Could you check a few things on this model? Use its own coordinates, in mm. A direction names the side the tool comes from. Round coordinates to 2 decimals unless told otherwise and drop trailing zeros. Write each loop counter-clockwise with the first axis right and the second up, starting at its lowest first coordinate (ties: lowest second). Pieces come first, ordered by that corner, then holes. Notation, with made-up numbers: (31, 89) -> (69, 89) arc R15 cw to (69, 104) -> close; hole circle Ø3 at (21, 45). An arc over 180 degrees is marked (long way). Answer in a Markdown table with one row per item. Add a question column.
```python
from build123d import *

# Parameters (mm, degrees)
SKETCH1_W                      = 75.565
SKETCH1_H                      = 35.56
BOSS_EXTRUDE1_DEPTH            = 3.175
SKETCH5_W                      = 12.7
SKETCH5_H                      = 3.175
BOSS_EXTRUDE3_DEPTH            = 14.986
SKETCH6_W                      = 3.175
SKETCH6_H                      = 9.028368652
BOSS_EXTRUDE4_DEPTH            = 14.986
BOSS_EXTRUDE5_DEPTH            = 12.7
BOSS_EXTRUDE6_DEPTH            = 9.028368652
BOSS_EXTRUDE7_DEPTH            = 75.565
SKETCH10_W                     = 75.565
SKETCH10_H                     = 23.368
BOSS_EXTRUDE8_DEPTH            = 5.08
CUT_EXTRUDE1_DEPTH             = 82.106081899
CUT_EXTRUDE2_REACH             = 52.218
SKETCH12_W                     = 6.35
SKETCH12_H                     = 3.175
CUT_EXTRUDE2_DIRECTION_2_DEPTH = 51.217629864
CUT_EXTRUDE3_DEPTH             = 55.104465738
CUT_EXTRUDE4_REACH             = 55.629
SKETCH14_W                     = 2.54
SKETCH14_H                     = 3.81


with BuildPart() as part:
    # Sketch1 → Boss-Extrude1 (new body)
    with BuildSketch(Plane.XY):
        Rectangle(SKETCH1_W, SKETCH1_H)
    extrude(amount=-BOSS_EXTRUDE1_DEPTH)

    # Sketch5 → Boss-Extrude3 (add)
    with BuildSketch(Plane.XY):
        with Locations((0, 16.1925)):
            Rectangle(SKETCH5_W, SKETCH5_H)
        with Locations((0, -16.1925)):
            Rectangle(SKETCH5_W, SKETCH5_H)
    extrude(amount=BOSS_EXTRUDE3_DEPTH)

    # Sketch6 → Boss-Extrude4 (add)
    with BuildSketch(Plane.XY):
        with Locations((-36.195, 0)):
            Rectangle(SKETCH6_W, SKETCH6_H)
        with Locations((36.195, 0)):
            Rectangle(SKETCH6_W, SKETCH6_H)
    extrude(amount=BOSS_EXTRUDE4_DEPTH)

    # Sketch7 → Boss-Extrude5 (add)
    with BuildSketch(Plane.ZY.offset(6.35)):
        Polygon((14.986, -17.78), (14.986, -11.43), (21.336, -17.78), align=None)
        Polygon((14.986, 17.78), (14.986, 11.43), (21.336, 17.78), align=None)
    extrude(amount=-BOSS_EXTRUDE5_DEPTH)

    # Sketch8 → Boss-Extrude6 (add)
    with BuildSketch(Plane.XZ.offset(4.514184326)):
        Polygon((-37.7825, 14.986), (-31.4325, 14.986), (-37.7825, 21.336), align=None)
        Polygon((37.7825, 14.986), (31.4325, 14.986), (37.7825, 21.336), align=None)
    extrude(amount=-BOSS_EXTRUDE6_DEPTH)

    # Sketch9 → Boss-Extrude7 (add)
    with BuildSketch(Plane.ZY.offset(37.7825)):
        Polygon((-3.175, 17.78), (-18.572931679, 8.89), (-3.175, -17.78), align=None)
    extrude(amount=-BOSS_EXTRUDE7_DEPTH)

    # Sketch10 → Boss-Extrude8 (add)
    with BuildSketch(Plane(origin=(0, -5.819815329, -10.08021584), x_dir=(-1, 0, 0), z_dir=(0, -0.5000000000000012, -0.866025403784438))):
        with Locations((0, -2.126431679)):
            Rectangle(SKETCH10_W, SKETCH10_H)
    extrude(amount=BOSS_EXTRUDE8_DEPTH)

    # Sketch11 → Cut-Extrude1 (cut, through all)
    with BuildSketch(Plane.ZY.offset(37.7825)):
        Polygon((-14.859, 2.457281636), (0, 4.514184326), (36.888684706, 18.275511072), (5.286071508, 25.150339228), (-30.3838484, 8.233222823), align=None)
        Polygon((-3.175, -17.78), (-8.125516688, -9.205453573), (0, -4.514184326), (40.158547499, -20.406390647), (15.599703883, -25.394905756), align=None)
    extrude(amount=-CUT_EXTRUDE1_DEPTH, mode=Mode.SUBTRACT)

    # Cut-Extrude2: up to this plane
    cut_extrude2_end = Plane(origin=(37.7825, -9.205453573, -8.125516688), z_dir=(0, 0.8660254037844387, -0.5))
    # Sketch12 → Cut-Extrude2 (cut, up to the surface)
    with BuildSketch(Plane(origin=(0, 4.429308453, -0.61314062), x_dir=(1, 0, 0), z_dir=(0, 0.9905543702216956, -0.13712052958875406)), mode=Mode.PRIVATE) as cut_extrude2_sk1:
        with Locations((0, 4.143512655)):
            Rectangle(SKETCH12_W, SKETCH12_H)
    cut_extrude2_tool1 = split(extrude(cut_extrude2_sk1.sketch, amount=-CUT_EXTRUDE2_REACH, mode=Mode.PRIVATE), bisect_by=cut_extrude2_end, keep=Keep.BOTH, mode=Mode.PRIVATE)
    add(cut_extrude2_tool1.solids().sort_by_distance((0, 3.861148, -4.717515))[0], mode=Mode.SUBTRACT)

    # Sketch12 → Cut-Extrude2 direction 2 (cut)
    with BuildSketch(Plane(origin=(0, 4.429308453, -0.61314062), x_dir=(1, 0, 0), z_dir=(0, 0.9905543702216956, -0.13712052958875406))):
        with Locations((0, 4.143512655)):
            Rectangle(SKETCH12_W, SKETCH12_H)
    extrude(amount=CUT_EXTRUDE2_DIRECTION_2_DEPTH, mode=Mode.SUBTRACT)

    # Sketch13 → Cut-Extrude3 (cut, through all)
    with BuildSketch(Plane(origin=(0, 8.277096964, -4.77878416), x_dir=(1, 0, 0), z_dir=(0, 0.866025403784438, -0.5000000000000012))):
        Polygon((-29.21, 11.639630657), (-37.7825, 0.917907837), (-37.7825, 11.639630657), (-37.7825, 16.719630657), (-29.21, 16.719630657), align=None)
        Polygon((37.7825, 0.917907837), (37.7825, 11.639630657), (37.7825, 16.719630657), (29.21, 16.719630657), (29.21, 11.639630657), align=None)
    extrude(amount=-CUT_EXTRUDE3_DEPTH, mode=Mode.SUBTRACT)

    # Sketch14 → Cut-Extrude4 (cut, up to next)
    with BuildSketch(Plane(origin=(0, -8.359815329, -14.479624891), x_dir=(-1, 0, 0), z_dir=(0, -0.5000000000000014, -0.8660254037844379)), mode=Mode.PRIVATE) as cut_extrude4_sk1:
        with Locations((-18.050542255, -5.844544168)):
            Rectangle(SKETCH14_W, SKETCH14_H)
    cut_extrude4_tool1 = extrude(cut_extrude4_sk1.sketch, amount=-CUT_EXTRUDE4_REACH, mode=Mode.PRIVATE) & part.part
    # Sketch14 → Cut-Extrude4 (cut, up to next)
    with BuildSketch(Plane(origin=(0, -8.359815329, -14.479624891), x_dir=(-1, 0, 0), z_dir=(0, -0.5000000000000014, -0.8660254037844379)), mode=Mode.PRIVATE) as cut_extrude4_sk2:
        with Locations((18.295855998, -5.844544168)):
            Rectangle(SKETCH14_W, SKETCH14_H)
    cut_extrude4_tool2 = extrude(cut_extrude4_sk2.sketch, amount=-CUT_EXTRUDE4_REACH, mode=Mode.PRIVATE) & part.part
    add(cut_extrude4_tool1.solids().sort_by_distance((18.050542, -13.421339, -11.557353))[0], mode=Mode.SUBTRACT)
    add(cut_extrude4_tool2.solids().sort_by_distance((-18.295856, -13.421339, -11.557353))[0], mode=Mode.SUBTRACT)


solid = part.part
```
(1) Suppose I cut it at C-C, the plane y = -3.75. Please give me the cut outline in (x, z) (1 decimal).
(2) Suppose I cut it at D-D, the plane z = -9. Please give me the cut outline in (x, y), then the cut area to 3 significant figures.
(3) I need wall thicknesses on L1, parallel to X at y = -12.5, z = -11.5; L2, parallel to X at y = -4, z = 5; L3, parallel to X at y = -7.75, z = -13.5. Which ranges of each line are inside material? Lowest first, please.
(4) If we mould it in two halves opening along Z, with no side actions, what happens to faces 1 (the face through (34.563, -0.063, 18.117)), 2 (the face through (33, 0, 14.986)), 3 (the face through (-19.566, -12, -9))? For each: pulls with the +Z half, pulls with the -Z half, needs draft (parallel to the pull), parting line crosses it, or undercut.
(5) Suppose I cut it at B-B, the plane z = 16.5. Please give me the cut outline in (x, y), then the cut area to 3 significant figures.
(6) On a 3-axis mill with a long thin cutter (end or side, diameter ignored), from which of +Z, -Z, +X, -X, +Y, -Y can I reach the whole of each face in a straight line? I mean faces 4 (the face through (-18.3, -13.8, -8.4)), 5 (the face through (19.321, -12, -9)), 6 (the face through (-33, 0, 14.986)). Say none if no direction works.
(7) For P1, Ø1.8, axis at y = -13.5, z = -10.5, coming from the +X side; P2, Ø13, axis at y = -9.5, z = -9.5, coming from the -X side; P3, Ø2, axis at x = 26, z = -11, coming from the -Y side; P4, Ø8, axis at y = -11, z = 4, coming from the -X side, each with a flat end and sliding along its axis, tell me the tip position at first contact or that it passes through.
(8) Suppose I cut it at A-A, the plane x = 18.5. Please give me the cut outline in (y, z) (3 decimals).
Response:
| question | item | result |
|---|---|---|
| 1 | outline | (-37.8, 1.1) -> (-29.2, -11.3) -> (-29.2, -17.1) -> (29.2, -17.1) -> (29.2, -11.3) -> (37.8, 1.1) -> (37.8, 21.3) -> (31.4, 15) -> (34.6, 15) -> (34.6, 0) -> (-34.6, 0) -> (-34.6, 15) -> (-31.4, 15) -> (-37.8, 21.3) -> close; hole (-3.2, -5.3) -> (3.2, -5.3) -> (3.2, -2.1) -> (-3.2, -2.1) -> close |
| 2 | outline | (-33.59, 3.27) -> (-29.21, -7.69) -> (-29.21, -17.85) -> (29.21, -17.85) -> (29.21, -7.69) -> (33.59, 3.27) -> close; hole (-19.57, -14.14) -> (-17.03, -14.14) -> (-17.03, -9.75) -> (-19.57, -9.75) -> close; hole (16.78, -14.14) -> (19.32, -14.14) -> (19.32, -9.75) -> (16.78, -9.75) -> close |
| 2 | area | 1,260 mm² |
| 3 | L1 | -29.21 to -19.57, -17.03 to 16.78, 19.32 to 29.21 |
| 3 | L2 | -37.78 to -34.61, 34.61 to 37.78 |
| 3 | L3 | -29.21 to 29.21 |
| 4 | face 1 | pulls with the +Z half |
| 4 | face 2 | undercut |
| 4 | face 3 | needs draft |
| 5 | outline | (-37.78, -4.51) -> (-32.95, -4.51) -> (-32.95, 4.51) -> (-37.78, 4.51) -> close; (32.95, -4.51) -> (37.78, -4.51) -> (37.78, 4.51) -> (32.95, 4.51) -> close |
| 5 | area | 87.3 mm² |
| 6 | face 4 | -Z |
| 6 | face 5 | none |
| 6 | face 6 | +Y, -Y |
| 7 | P1 | x = 29.21 |
| 7 | P2 | x = -33.34 |
| 7 | P3 | y = -16.12 |
| 7 | P4 | through |
| 8 | outline | (-20.32, -7.574) -> (-15.071, -10.605) -> (-12.531, -6.205) -> (-17.78, -3.175) -> close; (-11.772, -12.51) -> (-0.083, -19.258) -> (2.457, -14.859) -> (4.514, 0) -> (-4.514, 0) -> (-9.205, -8.126) -> (-9.232, -8.11) -> close |
